Drawing for the job (mm, zero at the part's lowest x, y, z). A direction names the side the tool comes from. Round coordinates to 2 decimals unless told otherwise and drop trailing zeros. Write each loop counter-clockwise with the first axis right and the second up, starting at its lowest first coordinate (ties: lowest second). Pieces come first, ordered by that corner, then holes. Notation, with made-up numbers: M 14,27 L 20,27 A5 ccw 20,35 Z; hole C -10,86 d7. An arc over 180 degrees is marked long. Use a Markdown table: item, result.
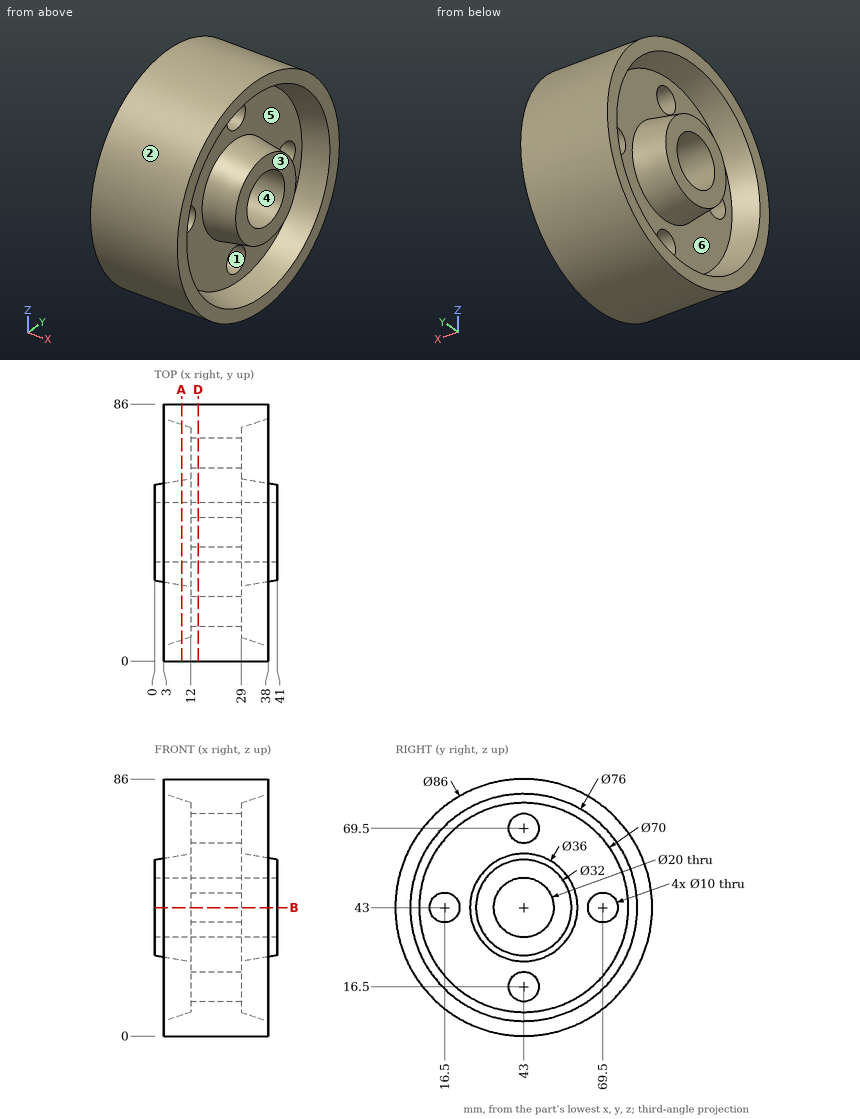
Q1. Which spindle directions (+Z, -Z, +X, -X, +Y, -Y) get a long thin tool onto all of the face, cutting with end or side? Do the marked faces 4, 5 and 6. Say none if no direction does.
Response values:
| item | result |
|---|---|
| face 4 | +X, -X |
| face 5 | +X |
| face 6 | -X |
Q2. Two-plate mould, pull along Z, no slides. Class the marked faces 1, 2 and 3: +Z half, -Z half, draft (parallel to the pull), parting line (faces both ways), or undercut.
Response values:
| item | result |
|---|---|
| face 1 | undercut |
| face 2 | parting line |
| face 3 | draft |
Q3. Cut at A-A on x = 9. Give the cut face in (y, z), and give its area (3 significant figures).
Response values:
| item | result |
|---|---|
| outline | C 43,43 d86; C 43,43 d35; hole C 43,43 d72; hole C 43,43 d20 |
| area | 2,390 mm2 |
Q4. Drill centre lines: L1, parallel to Y at x = 20.5, z = 38.5; L2, parallel to Z at x = 33.5, y = 45.5; L3, parallel to Z at x = 10.5, y = 34. Where is each one in solid material? Low to high.
Response values:
| item | result |
|---|---|
| L1 | y = 0.24 to 14.32, 18.68 to 34.07, 51.93 to 67.32, 71.68 to 85.76 |
| L2 | z = 0.07 to 6.59, 25.93 to 33.32, 52.68 to 60.07, 79.41 to 85.93 |
| L3 | z = 0.95 to 8.66, 27.7 to 38.64, 47.36 to 58.3, 77.34 to 85.05 |
Q5. Drop flat-ended pins along their axis: P1, Ø16, axis at y = 43, z = 69.5, coming from the -X side; P2, Ø2, axis at x = 14.5, y = 42, coming from the +Z side; P3, Ø3, axis at y = 48, z = 75, coming from the +X side; P4, Ø4, axis at y = 43, z = 18.5, coming from the -X side. Give the stop position or say it passes through.
Response values:
| item | result |
|---|---|
| P1 | stops at x = 12 |
| P2 | stops at z = 86 |
| P3 | stops at x = 29 |
| P4 | passes through |
Q6. Cut at B-B on z = 43. Count the separate pieces of the cut face and the enclosed holes in it, and give its area (3 significant figures).
Response values:
| item | result |
|---|---|
| separate pieces | 4 |
| enclosed holes | 0 |
| area | 1,350 mm2 |
Q7. Cut at D-D on x = 14.5. Give the cut face in (y, z), and give its area (3 significant figures).
Response values:
| item | result |
|---|---|
| outline | C 43,43 d86; hole C 16.5,43 d10; hole C 43,43 d20; hole C 43,16.5 d10; hole C 43,69.5 d10; hole C 69.5,43 d10 |
| area | 5,180 mm2 |
